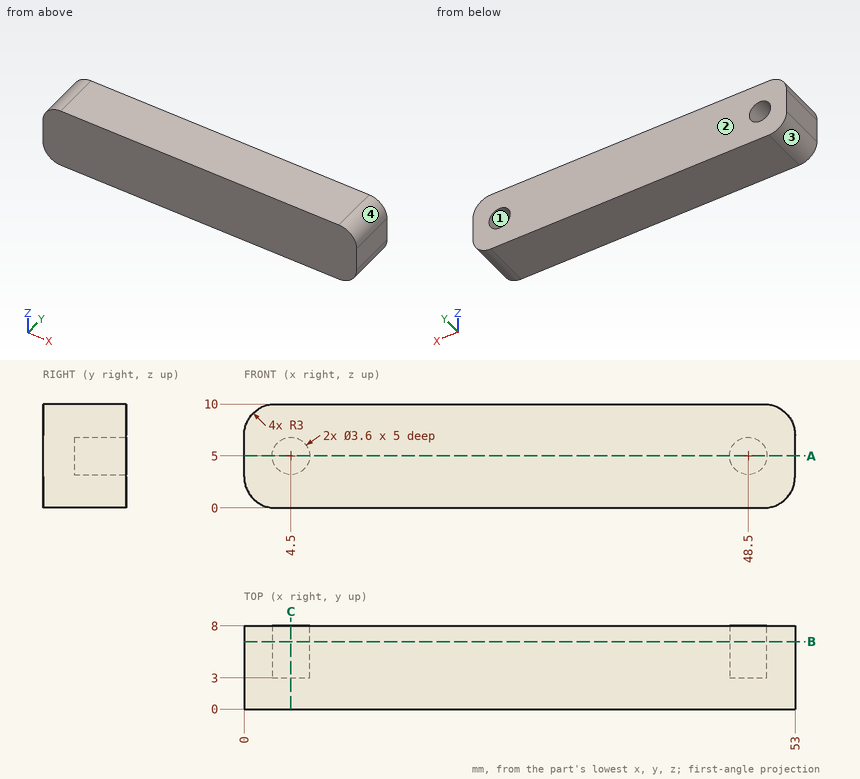
Study the drawing (mm; zero at the part's minimum x, y, z) and answer. Coordinates: 2 decimals unless noted, no trailing zeros. Write each loop counter-clockwise with the first axis right and the second up, starting at its lowest first coordinate (ties: lowest second). Pieces come first, ordered by that corner, then holes. Notation, with made-up numbers: M 19,56 L 24,56 A4 cw 24,60 Z; hole C 86,-20 d10. An arc over 180 degrees is marked long. Write each question's results on one line, items separated by ' | '.
Item 1: The part is cut by section B-B on y = 6.5. Determine the outline of the cut face in (x, z), and give its area (3 significant figures).
Answer below:
outline: M 0,3 A3 ccw 3,0 L 50,0 A3 ccw 53,3 L 53,7 A3 ccw 50,10 L 3,10 A3 ccw 0,7 Z; hole C 4.5,5 d3.6; hole C 48.5,5 d3.6 | area: 502 mm2
Item 2: Given P1, Ø1.1, axis at x = 48.5, z = 4.5, coming from the +Y side, flat-ended and moving along its own axis, determine where the tip first touches the part or whether it passes through.
Answer below:
P1: y = 3
Item 3: The part is cut by section C-C on x = 4.5. Determine the outline of the cut face in (y, z), and give its area (3 significant figures).
Answer below:
outline: M 0,0 L 8,0 L 8,3.2 L 3,3.2 L 3,6.8 L 8,6.8 L 8,10 L 0,10 Z | area: 62.0 mm2
Item 4: Consider probe 1 along Z at (x, y) = (48.5, 3.5); probe 2 along X at (y, z) = (5, 6); probe 3 along X at (y, z) = (3.25, 6.5). Determine where each line is inside the solid, lowest interval first. Write a range as [from, to].
Answer below:
probe 1: [0, 3.2], [6.8, 10] | probe 2: [0, 3], [6, 47], [50, 53] | probe 3: [0, 3.51], [5.49, 47.51], [49.49, 53]
Item 5: The part is cut by section A-A on z = 5. Determine the outline of the cut face in (x, y), and give its area (3 significant figures).
Answer below:
outline: M 0,0 L 53,0 L 53,8 L 50.3,8 L 50.3,3 L 46.7,3 L 46.7,8 L 6.3,8 L 6.3,3 L 2.7,3 L 2.7,8 L 0,8 Z | area: 388 mm2
Item 6: For a pull along X with two mould halves and no side action, classify the marked faces 1, 2, 3 and 4 as released by +X, released by -X, zero draft, split by the parting line, or undercut.
Answer below:
face 1: undercut | face 2: zero draft | face 3: released by -X | face 4: released by +X
